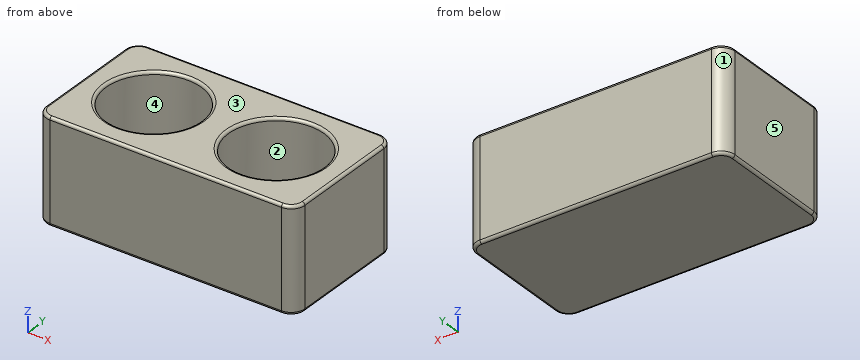
```python
from build123d import *

# Parameters (mm, degrees)
F0_W         = 95
F0_H         = 50
F0_R         = 17.5
F1_DEPTH     = 36
F2_W         = 95
F2_H         = 50
F3_DEPTH     = 2
F4_R         = 1
F5_T1_DEPTH  = 38
F5_T4_ANGLE  = 90
F5_T6_ANGLE  = 90
F5_T8_ANGLE  = 90
F5_T10_ANGLE = 90
F5_T12_ANGLE = 90
F5_T14_ANGLE = 90
F5_T16_ANGLE = 90
F5_T18_ANGLE = 90


# Not quite as in the source:
# - a fillet or chamfer that OpenCascade refuses, or shapes differently, is made with other operations: its cross-section is extruded or revolved along the edge and cut away or added


with BuildPart() as f1:
    # F0 (on Top) → F1 (new body)
    with BuildSketch(Plane.XY):
        Rectangle(F0_W, F0_H)
        with Locations((-22.5, 0)):
            Circle(F0_R, mode=Mode.SUBTRACT)
        with Locations((22.5, 0)):
            Circle(F0_R, mode=Mode.SUBTRACT)
    extrude(amount=F1_DEPTH)

    # F2 (on face) → F3 (join)
    with BuildSketch(Plane(origin=(0, 0, 0), x_dir=(1, 0, 0), z_dir=(0, 0, -1))):
        Rectangle(F2_W, F2_H)
    extrude(amount=F3_DEPTH)

    # F4
    f4_edges = [f1.edges().sort_by_distance(p)[0] for p in [
        (0, 25, 36),
        (-47.5, 0, 36),
        (0, -25, 36),
        (47.5, 0, 36),
        (-40, 0, 36),
        (5, 0, 36),
        (0, 25, -2),
        (47.5, 0, -2),
        (0, -25, -2),
        (-47.5, 0, -2),
    ]]
    fillet(f4_edges, radius=F4_R)

    # F5: fillet of radius 5 on 4 edges, made by hand

    # F5_s2 → F5_t1 (cut)
    with BuildSketch(Plane.XY.offset(-2)):
        with BuildLine():
            ThreePointArc((42.5, 25), (46.0355339059, 23.5355339059), (47.5, 20))
            Line((47.5, 20), (47.5, 25))
            Line((47.5, 25), (42.5, 25))
        make_face()
        with BuildLine():
            ThreePointArc((47.5, -20), (46.0355339059, -23.5355339059), (42.5, -25))
            Line((42.5, -25), (47.5, -25))
            Line((47.5, -25), (47.5, -20))
        make_face()
        with BuildLine():
            ThreePointArc((-47.5, -20), (-46.0355339059, -23.5355339059), (-42.5, -25))
            Line((-42.5, -25), (-47.5, -25))
            Line((-47.5, -25), (-47.5, -20))
        make_face()
        with BuildLine():
            ThreePointArc((-42.5, 25), (-46.0355339059, 23.5355339059), (-47.5, 20))
            Line((-47.5, 20), (-47.5, 25))
            Line((-47.5, 25), (-42.5, 25))
        make_face()
    extrude(amount=F5_T1_DEPTH, mode=Mode.SUBTRACT)

    # F5_s3 → F5_t4 (revolve, cut)
    with BuildSketch(Plane.XZ.offset(-20)):
        with BuildLine():
            ThreePointArc((-46.5, -2), (-47.2071067812, -1.7071067812), (-47.5, -1))
            Line((-47.5, -1), (-47.5, -2))
            Line((-47.5, -2), (-46.5, -2))
        make_face()
    revolve(axis=Axis((-42.5, 20, -2), (0, 0, -1)), revolution_arc=F5_T4_ANGLE, mode=Mode.SUBTRACT)

    # F5_s5 → F5_t6 (revolve, cut)
    with BuildSketch(Plane.YZ.offset(-42.5)):
        with BuildLine():
            ThreePointArc((24, 36), (24.7071067812, 35.7071067812), (25, 35))
            Line((25, 35), (25, 36))
            Line((25, 36), (24, 36))
        make_face()
    revolve(axis=Axis((-42.5, 20, 36), (0, 0, 1)), revolution_arc=F5_T6_ANGLE, mode=Mode.SUBTRACT)

    # F5_s7 → F5_t8 (revolve, cut)
    with BuildSketch(Plane.YZ.offset(-42.5)):
        with BuildLine():
            ThreePointArc((-24, -2), (-24.7071067812, -1.7071067812), (-25, -1))
            Line((-25, -1), (-25, -2))
            Line((-25, -2), (-24, -2))
        make_face()
    revolve(axis=Axis((-42.5, -20, -2), (0, 0, -1)), revolution_arc=F5_T8_ANGLE, mode=Mode.SUBTRACT)

    # F5_s9 → F5_t10 (revolve, cut)
    with BuildSketch(Plane.XZ.offset(20)):
        with BuildLine():
            ThreePointArc((-46.5, 36), (-47.2071067812, 35.7071067812), (-47.5, 35))
            Line((-47.5, 35), (-47.5, 36))
            Line((-47.5, 36), (-46.5, 36))
        make_face()
    revolve(axis=Axis((-42.5, -20, 36), (0, 0, 1)), revolution_arc=F5_T10_ANGLE, mode=Mode.SUBTRACT)

    # F5_s11 → F5_t12 (revolve, cut)
    with BuildSketch(Plane.YZ.offset(42.5)):
        with BuildLine():
            ThreePointArc((-24, 36), (-24.7071067812, 35.7071067812), (-25, 35))
            Line((-25, 35), (-25, 36))
            Line((-25, 36), (-24, 36))
        make_face()
    revolve(axis=Axis((42.5, -20, 36), (0, 0, 1)), revolution_arc=F5_T12_ANGLE, mode=Mode.SUBTRACT)

    # F5_s13 → F5_t14 (revolve, cut)
    with BuildSketch(Plane.XZ.offset(20)):
        with BuildLine():
            ThreePointArc((46.5, -2), (47.2071067812, -1.7071067812), (47.5, -1))
            Line((47.5, -1), (47.5, -2))
            Line((47.5, -2), (46.5, -2))
        make_face()
    revolve(axis=Axis((42.5, -20, -2), (0, 0, -1)), revolution_arc=F5_T14_ANGLE, mode=Mode.SUBTRACT)

    # F5_s15 → F5_t16 (revolve, cut)
    with BuildSketch(Plane.XZ.offset(-20)):
        with BuildLine():
            ThreePointArc((46.5, 36), (47.2071067812, 35.7071067812), (47.5, 35))
            Line((47.5, 35), (47.5, 36))
            Line((47.5, 36), (46.5, 36))
        make_face()
    revolve(axis=Axis((42.5, 20, 36), (0, 0, 1)), revolution_arc=F5_T16_ANGLE, mode=Mode.SUBTRACT)

    # F5_s17 → F5_t18 (revolve, cut)
    with BuildSketch(Plane.YZ.offset(42.5)):
        with BuildLine():
            ThreePointArc((24, -2), (24.7071067812, -1.7071067812), (25, -1))
            Line((25, -1), (25, -2))
            Line((25, -2), (24, -2))
        make_face()
    revolve(axis=Axis((42.5, 20, -2), (0, 0, -1)), revolution_arc=F5_T18_ANGLE, mode=Mode.SUBTRACT)


solid = f1.part
```
Model file for the job. Use its own axes, mm. Face numbers are marked on the shaded views. A direction names the side the tool comes from. Coordinates: 2 decimals unless noted, no trailing zeros. Loops run counter-clockwise (first coordinate to the right, second up) from the corner with the lowest first, then second, coordinate; pieces in that order, holes last. Notation, with made-up numbers: M -21.75,-5 L -7.75,-5 A23 cw -7.75,20 Z; hole C 66,63.25 d8. An arc over 180 degrees is marked long. Use CSV: the item, a comma, the result in double quotes. Start each with the question number.
1. Tool access for the marked faces 4 and 5: list every direction of +Z, -Z, +X, -X, +Y, -Y with a clear straight run to the whole face (end or side of a thin tool).
2. Band-saw the part on C-C, the plane y = 0. List the corners of the cut face in (x, z).
3. Flat gauge pin, fed straight in: pin 1 (21 mm diameter, centred on x = 22.5, y = 0, fed in from +Z). Where does the tip first touch, or does it go through?
4. Band-saw the part on B-B, the plane x = -22.5. List the corners of the cut face in (y, z), then the cut area to 3 significant figures.
5. Probe probe 1 along Y at (x, z) = (-22.5, 22); probe 2 along X at (y, z) = (-12, 20.5); probe 3 along X at (y, z) = (9, 15.5). List the from-to ranges inside material, lowest first. Write a range as [from, to].
6. Two-plate mould, pull along Y, no slides. Class the marked faces 1, 2 and 3: pulls with the +Y half, pulls with the -Y half, needs draft (parallel to the pull), parting line crosses it, or undercut.
7. Band-saw the part on A-A, the plane z = 13.5. List the corners of the cut face in (x, y).
Entries:
1,face 4,"+Z"
1,face 5,"+Z, -Z, -X, +Y, -Y"
2,outline,"M -47.5,-1 A1 ccw -46.5,-2 L 46.5,-2 A1 ccw 47.5,-1 L 47.5,35 A1 ccw 46.5,36 L 41,36 A1 ccw 40,35 L 40,0 L 5,0 L 5,35 A1 ccw 4,36 L -4,36 A1 ccw -5,35 L -5,0 L -40,0 L -40,35 A1 ccw -41,36 L -46.5,36 A1 ccw -47.5,35 Z"
3,pin 1,"stops at z = 0"
4,outline,"M -25,-1 A1 ccw -24,-2 L 24,-2 A1 ccw 25,-1 L 25,35 A1 ccw 24,36 L 18.5,36 A1 ccw 17.5,35 L 17.5,0 L -17.5,0 L -17.5,35 A1 ccw -18.5,36 L -24,36 A1 ccw -25,35 Z"
4,area,"639 mm2"
5,probe 1,"y = [-25, -17.5], [17.5, 25]"
5,probe 2,"x = [-47.5, -35.24], [-9.76, 9.76], [35.24, 47.5]"
5,probe 3,"x = [-47.5, -37.51], [-7.49, 7.49], [37.51, 47.5]"
6,face 1,"pulls with the +Y half"
6,face 2,"undercut"
6,face 3,"needs draft"
7,outline,"M -47.5,-20 A5 ccw -42.5,-25 L 42.5,-25 A5 ccw 47.5,-20 L 47.5,20 A5 ccw 42.5,25 L -42.5,25 A5 ccw -47.5,20 Z; hole C -22.5,0 d35; hole C 22.5,0 d35"
